Source: CAD feature listing. Evaluate the final solid. Frame: model axes, mm. A direction names the side the tool comes from. Give positions to 0.01 mm unless a question says otherwise; leave off trailing zeros. Loops run counter-clockwise (first coordinate to the right, second up) from the corner with the lowest first, then second, coordinate; pieces in that order, holes last. Notation, with made-up numbers: (26, -1) -> (43, -1) arc R19 cw to (43, 9) -> close; hole circle Ø10 at (14, 53.5). An arc over 180 degrees is marked (long way). Put each result on its own line as item: value.
```python
from build123d import *

# Parameters (mm, degrees)
SM_BASE_FLANGE_1_DEPTH = 5
OTHER_START            = -100.2
OTHER_1_OUTLINE_W      = 5.4
OTHER_1_OUTLINE_H      = 5
OTHER_1_DEPTH          = 20.4
OTHER_START_2          = -63.368595269
OTHER_1_2_OUTLINE_W    = 5.4
OTHER_1_2_OUTLINE_H    = 5
OTHER_1_2_DEPTH        = 20.4
OTHER_START_3          = -26.537190538
OTHER_1_3_OUTLINE_W    = 5.4
OTHER_1_3_OUTLINE_H    = 5
OTHER_1_3_DEPTH        = 20.4


# Read off the part's stored shape, not the designer's step: Выступы и прорези-Прорезь1
# Sheet-metal steps are written as plain solids
with BuildPart() as part:
    # Sketch 1 → Базовая кромка1 (new body)
    with BuildSketch(Plane.XY):
        with BuildLine():
            Line((-105, 0), (-105, 30))
            Line((-105, 30), (0.750859603, 103.635517522))
            Line((0.750859603, 103.635517522), (-1.337190538, 90.452087776))
            Line((-1.337190538, 90.452087776), (-1.337190538, 64.447388282))
            Line((-1.337190538, 64.447388282), (-28.337190538, 64.447388282))
            ThreePointArc((-28.337190538, 64.447388282), (-30.458510882, 63.568708625), (-31.337190538, 61.447388282))
            Line((-31.337190538, 61.447388282), (-31.337190538, 37.447388282))
            ThreePointArc((-31.337190538, 37.447388282), (-30.458510882, 35.326067938), (-28.337190538, 34.447388282))
            Line((-28.337190538, 34.447388282), (-1.337190538, 34.447388282))
            Line((-1.337190538, 34.447388282), (-1.337190538, 8.442688787))
            Line((-1.337190538, 8.442688787), (11.55423155, -72.950546947))
            Line((11.55423155, -72.950546947), (-14.065019195, -81.274746116))
            ThreePointArc((-14.065019195, -81.274746116), (-15.810987784, -82.765944166), (-15.991137761, -85.054966648))
            Line((-15.991137761, -85.054966648), (-8.574729896, -107.88032304))
            ThreePointArc((-8.574729896, -107.88032304), (-7.083531846, -109.626291629), (-4.794509364, -109.806441605))
            Line((-4.794509364, -109.806441605), (20.884016576, -101.462982757))
            Line((20.884016576, -101.462982757), (34.59610485, -143.664451098))
            ThreePointArc((34.59610485, -143.664451098), (33.691279446, -146.872719978), (30.380963802, -147.264521653))
            Line((30.380963802, -147.264521653), (5.64897556, -134.662944227))
            ThreePointArc((5.64897556, -134.662944227), (-7.242640853, -123.621288585), (-19.285450277, -111.659571558))
            Line((-19.285450277, -111.659571558), (-105, -20))
            Line((-105, -20), (-105, 0))
        make_face()
    extrude(amount=SM_BASE_FLANGE_1_DEPTH)

    # Other 1 outline → Other 1 (cut)
    with BuildSketch(Plane.YZ.offset(OTHER_START)):
        with Locations((-2.5, 2.5)):
            Rectangle(OTHER_1_OUTLINE_W, OTHER_1_OUTLINE_H)
    other_1 = extrude(amount=OTHER_1_DEPTH, mode=Mode.SUBTRACT)

    # Other 1 2 outline → Other 1 2 (cut)
    with BuildSketch(Plane.YZ.offset(OTHER_START_2)):
        with Locations((-2.5, 2.5)):
            Rectangle(OTHER_1_2_OUTLINE_W, OTHER_1_2_OUTLINE_H)
    other_1_2 = extrude(amount=OTHER_1_2_DEPTH, mode=Mode.SUBTRACT)

    # Other 1 3 outline → Other 1 3 (cut)
    with BuildSketch(Plane.YZ.offset(OTHER_START_3)):
        with Locations((-2.5, 2.5)):
            Rectangle(OTHER_1_3_OUTLINE_W, OTHER_1_3_OUTLINE_H)
    other_1_3 = extrude(amount=OTHER_1_3_DEPTH, mode=Mode.SUBTRACT)

    # Зеркальное отражение1: Other 1, Other 1 2, Other 1 3 across plane
    add(other_1.mirror(Plane.ZX.offset(12.5)), mode=Mode.SUBTRACT)
    add(other_1_2.mirror(Plane.ZX.offset(12.5)), mode=Mode.SUBTRACT)
    add(other_1_3.mirror(Plane.ZX.offset(12.5)), mode=Mode.SUBTRACT)


solid = part.part
```
(1) Section B-B on z = 3.65. Give the number of separate pieces and of enclosed holes in the cut face, then the cut area to 3 significant figures.
Calculated:
separate pieces: 1
enclosed holes: 6
area: 14,300 mm²
(2) Draft query along Y for faces 1 (the flat face through (-52.865, 66.302, 2.465)), 2 (the flat face through (-6.137, -3, 3)), 3 (the flat face through (-105, 5, 2)), 4 (the flat face through (-61.543, -66.471, 2.465)). Return one class per face: released by +Y, released by -Y, zero draft, split by the parting line, or undercut.
Calculated:
face 1: released by +Y
face 2: undercut
face 3: zero draft
face 4: released by -Y
(3) Line query: probe 1 along Y at (x, z) = (-3.5, 3.65); probe 2 along Y at (x, z) = (-25, 0.35); probe 3 along Y at (x, z) = (-26.5, 1.5). Output: solid intervals per line, ascending. Write a range as from..to.
Calculated:
probe 1: y = -127..-109.39, -77.84..34.45, 64.45..100.68
probe 2: y = -105.55..-5.2, 0.2..24.8, 30.2..34.45, 64.45..85.7
probe 3: y = -103.94..-5.2, 0.2..24.8, 30.2..34.45, 64.45..84.66
(4) Section A-A on x = -23. Return loops of the section in (y, z).
Calculated:
outline: (-107.69, 0) -> (-5.2, 0) -> (-5.2, 5) -> (-107.69, 5) -> close; (0.2, 0) -> (24.8, 0) -> (24.8, 5) -> (0.2, 5) -> close; (30.2, 0) -> (34.45, 0) -> (34.45, 5) -> (30.2, 5) -> close; (64.45, 0) -> (87.1, 0) -> (87.1, 5) -> (64.45, 5) -> close
(5) Section C-C on y = 16. Return loops of the section in (x, z), then the cut area to 3 significant figures.
Calculated:
outline: (-105, 0) -> (-1.34, 0) -> (-1.34, 5) -> (-105, 5) -> close
area: 518 mm²
(6) First-contact query: P1, Ø2.5, axis at x = -14.5, z = 2, coming from the -Y side; P2, Ø1, axis at y = 50.5, z = 2.5, coming from the -X side; P3, Ø1.5, axis at x = -13, z = 1.5, coming from the +Y side. Flat tips, straight axial feed; report the tip coordinate or a pass-through.
Calculated:
P1: stops at y = -117.87
P2: stops at x = -76.28
P3: stops at y = 94.58
(7) Reachability of faces 5 (the flat face through (-90, 0.2, 2)), 6 (the flat face through (-1.337, 22, 2)), 7 (the flat face through (18.188, -141.052, 2.465)) from +Z, -Z, +X, -X, +Y, -Y: full face, straight path, thin tool, end or side. Return the list, or none.
Calculated:
face 5: +Z, -Z
face 6: +Z, -Z, +X
face 7: +Z, -Z, -X, -Y
(8) Section D-D on x = -76. Return loops of the section in (y, z), then the cut area to 3 significant figures.
Calculated:
outline: (-51.01, 0) -> (50.19, 0) -> (50.19, 5) -> (-51.01, 5) -> close
area: 506 mm²
